Autodesk Fusion 360 part; units mm, degrees
sketch "Sketch1" plane through (0, 0, 0) normal (0, 1, 0) x (1, 0, 0)
  line L0 (0, 0) -> (25, 0)
  line L1 (25, 0) -> (25, -10)
  line L2 (25, -10) -> (0, -10)
  line L3 (0, -10) -> (0, 0)
  line L4 (0, -10) -> (10, -10)
  line L5 (25, 0) -> (15, 0)
  line L6 (0, 0) -> (10, -10)
  line L7 (15, 0) -> (25, -10)
  circle A0 centre (5, -5) radius 1.5
  circle A1 centre (20, -5) radius 1.5
  dimension "d1" = 25
  dimension "d2" = 10
  dimension "d3" = 10
  dimension "d4" = 10
  dimension "d5" = 3
  dimension "d6" = 3
extrude "Extrude1" add sketch "Sketch1" against normal blind 2
extrude "Extrude2" add sketch "Sketch1" along normal blind 15 contours L6 A0 | L6 A0 | L7 A1 | L7 A1
Read the model definition and answer for the solid it produces. Units are mm, in the model's axes. A direction names the side the tool comes from. Give positions to 0.01 mm unless a question says otherwise; leave off trailing zeros. Write each loop counter-clockwise with the first axis right and the second up, starting at its lowest first coordinate (ties: lowest second). Pieces come first, ordered by that corner, then holes. Notation, with made-up numbers: (28.5, 39.5) -> (36.5, 39.5) arc R9 ccw to (36.5, 51.5) -> close; hole circle Ø8 at (71.25, 0.5). An arc over 180 degrees is marked (long way). Answer as a JSON object with one key per item and string values. Group by question number.
1) The mould has two halves that part along X. Classify faces 3 (the cylindrical face through (6.386, 7.395, 4.425)), 4 (the flat face through (25, -1, 5)), 5 (the flat face through (5, 15, 5)): +X half, -X half, draft (parallel to the pull), parting line (faces both ways), or undercut.
2) Find section C-C (z = 5). Write down the section's boundary in (x, y).
3) Find section B-B (y = 11.75). Write down the section's boundary in (x, z), and give its area (3 significant figures).
4) Consider L1, parallel to X at y = 7, z = 4; L2, parallel to Y at x = 5.5, z = 1; L3, parallel to X at y = 8.75, z = 4.5. Determine where each line is inside the solid, lowest interval first. Write a range as from..to.
5) Find section A-A (x = 20). Write down the section's boundary in (y, z).
6) A tool of negligible diameter and unlimited length cuts with its end or side. For faces 1 (the flat face through (0, -1, 5)), 2 (the cylindrical face through (18.5, 7.4, 5.07)), from which of +Z, -Z, +X, -X, +Y, -Y can it reach the whole face along a straight path? Write none if from no direction.
7) Find section D-D (z = 2.75). Write down the section's boundary in (x, y), and give its area (3 significant figures).
8) Each of these flat-tipped pins is pushed along its axis until it touches: P1, Ø10, axis at x = 7.5, y = 11, coming from the +Z side; P2, Ø1.5, axis at x = 20.5, z = 8.5, coming from the +Y side; P3, Ø6, axis at y = 7.5, z = 9, coming from the -X side. Where does it stop, or does it pass through?
Values follow:
{
 "1": {"face 3": "undercut", "face 4": "+X half", "face 5": "draft"},
 "2": {"outline": "(0, -2) -> (25, -2) -> (25, 0) -> (21.5, 0) -> (21.5, 15) -> (18.5, 15) -> (18.5, 0) -> (6.5, 0) -> (6.5, 15) -> (3.5, 15) -> (3.5, 0) -> (0, 0) -> close"},
 "3": {"outline": "circle Ø3 at (5, 5); circle Ø3 at (20, 5)", "area": "14.1 mm2"},
 "4": {"L1": "x = 3.88..6.12, 18.88..21.12", "L2": "y = -2..0", "L3": "x = 3.59..6.41, 18.59..21.41"},
 "5": {"outline": "(-2, 0) -> (0, 0) -> (0, 3.5) -> (15, 3.5) -> (15, 6.5) -> (0, 6.5) -> (0, 10) -> (-2, 10) -> close"},
 "6": {"face 1": "+Z, -Z, -X, +Y, -Y", "face 2": "+Y"},
 "7": {"outline": "(0, -2) -> (25, -2) -> (25, 0) -> (0, 0) -> close", "area": "50.0 mm2"},
 "8": {"P1": "stops at z = 6.5", "P2": "stops at y = 0", "P3": "stops at x = 3.88"}
}
